For this review, take the finished solid that the model builds, in its own axes (mm). Face numbers are marked on the shaded views. A direction names the side the tool comes from. Coordinates: 2 decimals unless noted, no trailing zeros. Write each loop counter-clockwise with the first axis right and the second up, starting at its lowest first coordinate (ties: lowest second). Pieces come first, ordered by that corner, then holes. Notation, with made-up numbers: M -13.75,20.25 L 27.25,20.25 A23 ccw 27.25,36.25 Z; hole C -18,47.5 d1. An arc over 180 degrees is marked long. One line per question, with ' | ' between items.
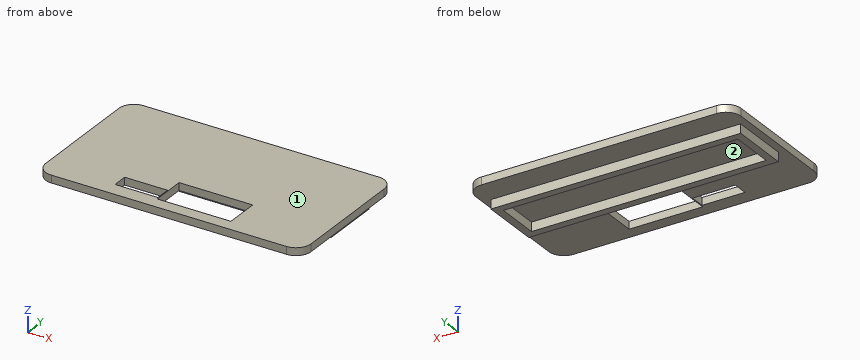
from build123d import *

# Parameters (mm, degrees)
F0_W     = 52.6
F0_H     = 28.8
F0_W_2   = 49.5
F0_H_2   = 11.8
F0_W_3   = 48
F0_H_3   = 2.52
F0_W_4   = 46.5
F0_H_4   = 8.8
F0_W_5   = 8.5
F0_H_5   = 3
F0_W_6   = 46.4
F0_H_6   = 0.92
F1_DEPTH = 1.5
F2_DEPTH = 1.8
F3_R     = 3


with BuildPart() as f1:
    # F0 (on Top) → F1 (new body)
    with BuildSketch(Plane.XY):
        with Locations((-2.8558062509, 6.2837967607)):
            Rectangle(F0_W, F0_H)
        Polygon((-26.6058062509, -3.4749299184), (-22.0043773293, -3.4749299184), (-22.0043773293, 1.2337967607), (20.8956226707, 1.2337967607), (20.8956226707, -4.7466191463), (20.8941937491, -4.7466191463), (20.8941937491, -5.2662032393), (20.8941937491, -5.8827909378), (20.8941937491, -6.0662032393), (-26.6058062509, -6.0662032393), (-26.6058062509, -5.2662032393), align=None, mode=Mode.SUBTRACT)
        with Locations((-2.9058062509, 9.5737967607)):
            Rectangle(F0_W_2, F0_H_2, mode=Mode.SUBTRACT)
        with Locations((-2.6558062509, 17.6337967607)):
            Rectangle(F0_W_3, F0_H_3, mode=Mode.SUBTRACT)
        with Locations((-2.9058062509, 9.5737967607)):
            Rectangle(F0_W_2, F0_H_2)
        with Locations((-2.9058062509, 9.5737967607)):
            Rectangle(F0_W_4, F0_H_4, mode=Mode.SUBTRACT)
        with Locations((-2.9058062509, 9.5737967607)):
            Rectangle(F0_W_4, F0_H_4)
        Polygon((-22.0043773293, 1.2337967607), (-22.0043773293, -3.4749299184), (-26.6058062509, -3.4749299184), (-26.6058062509, -5.2662032393), (-26.6058062509, -6.0662032393), (20.8941937491, -6.0662032393), (20.8941937491, -5.8827909378), (20.8941937491, -5.2662032393), (20.8941937491, -4.7466191463), (20.8956226707, -4.7466191463), (20.8956226707, 1.2337967607), align=None)
        with Locations((-11.1558062509, -3.6662032393)):
            Rectangle(F0_W_5, F0_H_5, mode=Mode.SUBTRACT)
        Polygon((7.8941937491, 1.1337967607), (7.8941937491, -5.2662032393), (7.8941937491, -5.3662032393), (20.7941937491, -5.3662032393), (20.7941937491, -5.9662032393), (-26.5058062509, -5.9662032393), (-26.5058062509, -5.3662032393), (-6.7058062509, -5.3662032393), (-6.7058062509, -5.2662032393), (-6.7058062509, 1.1337967607), align=None, mode=Mode.SUBTRACT)
        with Locations((-2.6558062509, 17.6337967607)):
            Rectangle(F0_W_3, F0_H_3)
        with Locations((-2.6558062509, 17.6337967607)):
            Rectangle(F0_W_6, F0_H_6, mode=Mode.SUBTRACT)
        with Locations((-2.6558062509, 17.6337967607)):
            Rectangle(F0_W_6, F0_H_6)
        Polygon((20.7941937491, -5.3662032393), (7.8941937491, -5.3662032393), (7.8941937491, -5.6662032393), (-6.7058062509, -5.6662032393), (-6.7058062509, -5.3662032393), (-26.5058062509, -5.3662032393), (-26.5058062509, -5.9662032393), (20.7941937491, -5.9662032393), align=None)
    extrude(amount=F1_DEPTH)

    # F0 (on Top) → F2 (join)
    with BuildSketch(Plane.XY):
        with Locations((-2.9058062509, 9.5737967607)):
            Rectangle(F0_W_2, F0_H_2)
        with Locations((-2.9058062509, 9.5737967607)):
            Rectangle(F0_W_4, F0_H_4, mode=Mode.SUBTRACT)
    extrude(amount=-F2_DEPTH)

    # F3
    f3_edges = [f1.edges().sort_by_distance(p)[0] for p in [
        (23.444194, -8.116203, 0.75),
        (23.444194, 20.683797, 0.75),
        (-29.155806, 20.683797, 0.75),
        (-29.155806, -8.116203, 0.75),
    ]]
    fillet(f3_edges, radius=F3_R)


solid = f1.part
1. Clearance check with flat-ended pins moving along their axes: P1, Ø10, axis at x = 18, y = -1.5, coming from the -Z side; P2, Ø0.9, axis at y = 7.5, z = -1.5, coming from the +X side; P3, Ø0.9, axis at x = -8, z = -1, coming from the +Y side. State where each tip first meets the part, or that it passes through.
Computed values:
P1: stops at z = 0 | P2: stops at x = 21.84 | P3: stops at y = 15.47
2. For line 1 along X through (y, z) = (-2.75, 0.8); line 2 along Y through (x, z) = (9, -0.95); line 3 along Z through (x, y) = (-8.5, 6.25), list the stretches that pass through material, from the lowest coordinate up.
Computed values:
line 1: x = -29.16 to -15.41, -6.91 to -6.71, 7.89 to 23.44 | line 2: y = 3.67 to 5.17, 13.97 to 15.47 | line 3: z = 0 to 1.5
3. Take a section at A-A on x = 0. State the section outline as (y, z) points.
Computed values:
outline: M -8.12,0 L -5.67,0 L -5.67,1.5 L -8.12,1.5 Z; M 1.13,0 L 3.67,0 L 3.67,-1.8 L 5.17,-1.8 L 5.17,0 L 13.97,0 L 13.97,-1.8 L 15.47,-1.8 L 15.47,0 L 20.68,0 L 20.68,1.5 L 1.13,1.5 Z
4. Take a section at B-B on z = -1.15. State the section outline as (x, y) points, plus the area to 3 significant figures.
Computed values:
outline: M -27.66,3.67 L 21.84,3.67 L 21.84,15.47 L -27.66,15.47 Z; hole M -26.16,5.17 L 20.34,5.17 L 20.34,13.97 L -26.16,13.97 Z | area: 175 mm2
5. Take a section at D-D on y = 14.5. State the section outline as (x, z) points.
Computed values:
outline: M -29.16,0 L -27.66,0 L -27.66,-1.8 L 21.84,-1.8 L 21.84,0 L 23.44,0 L 23.44,1.5 L -29.16,1.5 Z
6. Take a section at C-C on y = -2.75. State the section outline as (x, z) points, plus the area to 4 significant figures.
Computed values:
outline: M -29.16,0 L -15.41,0 L -15.41,1.5 L -29.16,1.5 Z; M -6.91,0 L -6.71,0 L -6.71,1.5 L -6.91,1.5 Z; M 7.89,0 L 23.44,0 L 23.44,1.5 L 7.89,1.5 Z | area: 44.25 mm2
7. Machinability: for the marked faces 1 and 2, which of the approach directions +Z, -Z, +X, -X, +Y, -Y give a long, thin tool a straight path to every point of the face, cutting with its end or side? Answer none if there is none.
Computed values:
face 1: +Z, +X, -X, +Y, -Y | face 2: -Z
